```python
from build123d import *

# Parameters (mm, degrees)
CROQUIS1_R              = 3.175
SALIENTE_EXTRUIR1_DEPTH = 6.35


with BuildPart() as part:
    # Croquis1 → Saliente-Extruir1 (new, symmetric)
    with BuildSketch(Plane.XY):
        with BuildLine():
            Line((30, 10), (30, 0))
            Line((30, 0), (-30, 0))
            Line((-30, 0), (-30, 10))
            ThreePointArc((-30, 10), (0, 40), (30, 10))
        make_face()
        with Locations((0, 10)):
            Circle(CROQUIS1_R, mode=Mode.SUBTRACT)
    extrude(amount=SALIENTE_EXTRUIR1_DEPTH, both=True)


solid = part.part
```
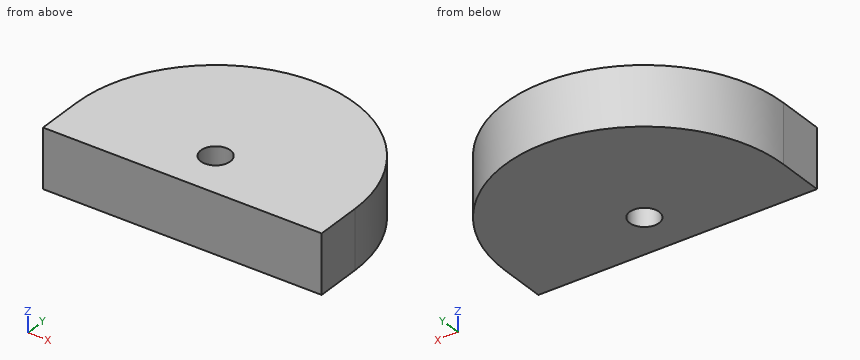
Input: part model. Units: mm. Frame: model coordinates. Give positions to 0.01 mm unless a question says otherwise; leave off trailing zeros. Order: outer loops, then holes, each group sorted by start corner. A loop starts at its lowest first (then second) coordinate and runs counter-clockwise, first axis right, second up.
1. Material intervals for L1, parallel to Y at x = 0, z = -2 (3 decimals); L2, parallel to X at y = 10.5, z = 2.25; L3, parallel to X at y = 29, z = 1, sorted ascending.
Derived:
L1: y = 0 to 6.825, 13.175 to 40
L2: x = -30 to -3.14, 3.14 to 30
L3: x = -23.22 to 23.22
2. Section C-C on y = 24. Return the cut outline in (x, z), and give its area (3 significant figures).
Derived:
outline: (-26.53, -6.35) - (26.53, -6.35) - (26.53, 6.35) - (-26.53, 6.35) - close
area: 674 mm2
3. Section B-B on z = 2.25. Return the cut outline in (x, y) (3 decimals), and give its area (3 significant figures).
Derived:
outline: (-30, 0) - (30, 0) - (30, 10) arc R30 ccw to (-30, 10) - close; hole circle Ø6.35 at (0, 10)
area: 1,980 mm2
4. Pin query (flat end, axial travel): pin 1 (1 mm diameter, centred on y = 24, z = -4.5, fed in from +X); pin 2 (4 mm diameter, centred on x = 5, z = -1, fed in from +Y). Return the tip coordinate at first contact, or that it passes through.
Derived:
pin 1: stops at x = 26.79
pin 2: stops at y = 39.85
5. Section A-A on x = 0. Return the cut outline in (y, z) (3 decimals), and give its area (3 significant figures).
Derived:
outline: (0, -6.35) - (6.825, -6.35) - (6.825, 6.35) - (0, 6.35) - close; (13.175, -6.35) - (40, -6.35) - (40, 6.35) - (13.175, 6.35) - close
area: 427 mm2
6. Section D-D on x = 23. Return the cut outline in (y, z), and give its area (3 significant figures).
Derived:
outline: (0, -6.35) - (29.26, -6.35) - (29.26, 6.35) - (0, 6.35) - close
area: 372 mm2
